from build123d import *

# Parameters (mm, degrees)
BOSS_EXTRUDE1_DEPTH        = 20
F_10_CLEARANCE_HOLE1_D     = 4.9784
F_10_CLEARANCE_HOLE1_DEPTH = 29.83
F_10_CLEARANCE_HOLE1_TIP   = 1.495662253


with BuildPart() as part:
    # Sketch2 → Boss-Extrude1 (new body, symmetric)
    with BuildSketch(Plane(origin=(0, 0, 0), x_dir=(0, 0, -1), z_dir=(1, 0, 0))):
        with BuildLine():
            Line((0, 20), (0, 0))
            ThreePointArc((0, 0), (5, -5), (10, 0))
            Line((10, 0), (10, 20))
            Line((10, 20), (0, 20))
        make_face()
    extrude(amount=BOSS_EXTRUDE1_DEPTH, both=True)

    # #10 Clearance Hole1
    with Locations(Plane.XY):
        with Locations((-14, 11.5), (14, 11.5)):
            Hole(F_10_CLEARANCE_HOLE1_D / 2, depth=F_10_CLEARANCE_HOLE1_DEPTH)
            with Locations((0, 0, -(F_10_CLEARANCE_HOLE1_DEPTH + F_10_CLEARANCE_HOLE1_TIP / 2))):  # 118° drill point
                Cone(0, F_10_CLEARANCE_HOLE1_D / 2, F_10_CLEARANCE_HOLE1_TIP, mode=Mode.SUBTRACT)


solid = part.part
The model under review builds one solid part; all positions refer to its coordinate system, in mm. Round coordinates to 2 decimals unless told otherwise and drop trailing zeros. Loops run counter-clockwise (first coordinate to the right, second up) from the corner with the lowest first, then second, coordinate; pieces in that order, holes last. Notation, with made-up numbers: (32.25, -7) -> (49.25, -7) arc R24 ccw to (49.25, 16) -> close; hole circle Ø6 at (-17, -2.5). An arc over 180 degrees is marked (long way). One line per question, with ' | ' between items. Start each with the question number.
Item 1: Draft analysis for pull direction X (two halves, no side actions). For faces 1 (the face through (12.851, 9.292, -5.07)), 2 (the face through (-20, 8, -5)), 3 (the face through (20, 8, -5)), state which applies: +X half, -X half, draft (parallel to the pull), parting line (faces both ways), or undercut.
Item 2: Add section B-B, the plane x = 14. Write out the cut boundary in (y, z), then the cut area to 3 significant figures.
Item 3: Add section A-A, the plane y = 11.5. Write out the cut boundary in (x, z).
Item 4: Add section D-D, the plane x = -6. Write out the cut boundary in (y, z).
Item 5: Add section C-C, the plane z = -5. Write out the cut boundary in (x, y).
Item 6: Wall thickness on line 1 along X through (y, z) = (10, -2.25); line 2 along X through (y, z) = (13.75, -5.5); line 3 along Y through (x, z) = (14, -7.5): over which ranges is each line inside the solid? List them lowest first. Write a range as [from, to].
Return value:
1) face 1: undercut | face 2: -X half | face 3: +X half
2) outline: (0, -10) -> (9.01, -10) -> (9.01, 0) -> (0, 0) arc R5 ccw to start; (13.99, -10) -> (20, -10) -> (20, 0) -> (13.99, 0) -> close | area: 189 mm2
3) outline: (-20, -10) -> (-16.49, -10) -> (-16.49, 0) -> (-20, 0) -> close; (-11.51, -10) -> (11.51, -10) -> (11.51, 0) -> (-11.51, 0) -> close; (16.49, -10) -> (20, -10) -> (20, 0) -> (16.49, 0) -> close
4) outline: (0, -10) -> (20, -10) -> (20, 0) -> (0, 0) arc R5 ccw to start
5) outline: (-20, -5) -> (20, -5) -> (20, 20) -> (-20, 20) -> close; hole circle Ø4.98 at (-14, 11.5); hole circle Ø4.98 at (14, 11.5)
6) line 1: x = [-20, -15.99], [-12.01, 12.01], [15.99, 20] | line 2: x = [-20, -15.06], [-12.94, 12.94], [15.06, 20] | line 3: y = [-4.33, 9.01], [13.99, 20]
